Print and shaded views of the part. All mm, measured from the part's lowest x, y and z. Give positions to 0.01 mm unless a question says otherwise; leave off trailing zeros. Loops run counter-clockwise (first coordinate to the right, second up) from the corner with the lowest first, then second, coordinate; pieces in that order, holes last.
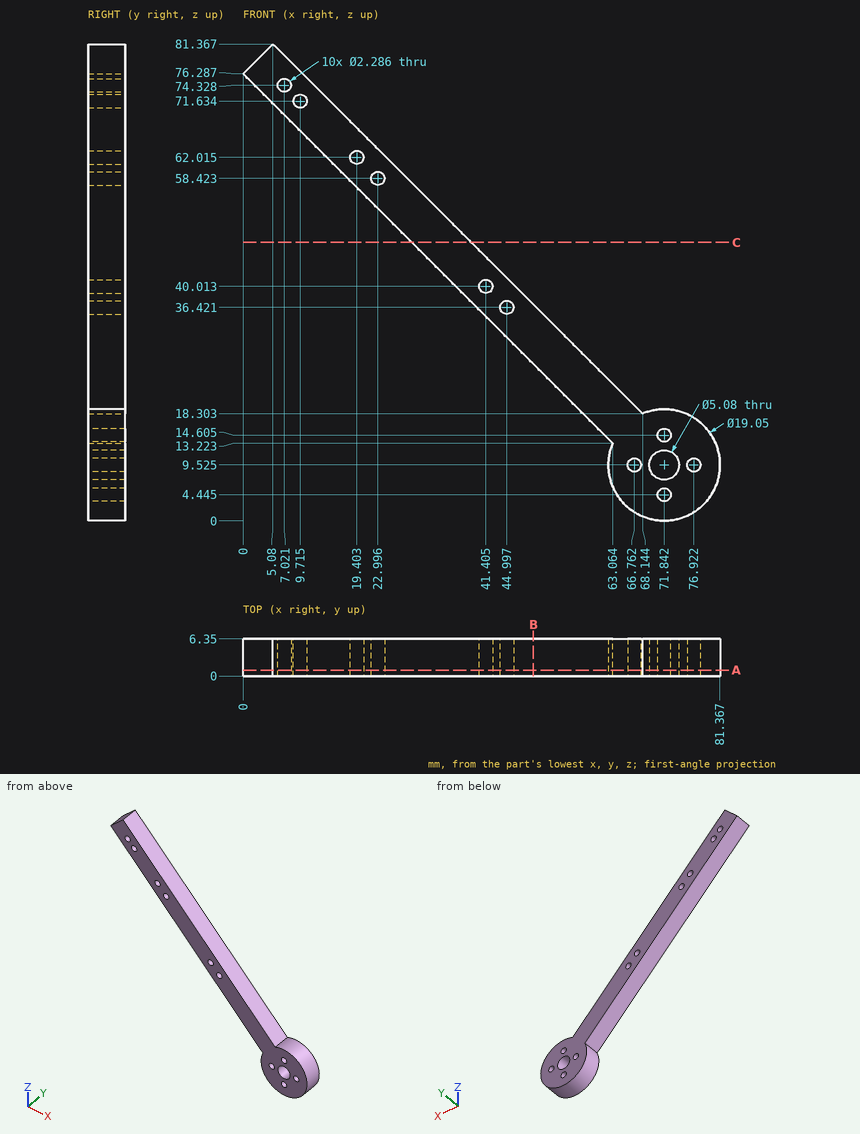
1. Probe line 1 along X through (y, z) = (5.5, 10.5) (1 decimal); line 2 along X through (y, z) = (4, 10) (1 decimal); line 3 along Z through (x, y) = (45, 6) (1 decimal). List the from-to ranges inside material, lowest first.
Responses:
line 1: x = 62.4 to 66.2, 67.4 to 69.5, 74.2 to 76.3, 77.5 to 81.3
line 2: x = 62.3 to 65.7, 67.8 to 69.3, 74.3 to 75.9, 78 to 81.4
line 3: z = 31.3 to 35.3, 37.6 to 41.4
2. Drop flat-ended pins along their axis: pin 1 (3 mm diameter, centred on x = 16, y = 2, fed in from +Z); pin 2 (3 mm diameter, centred on y = 3, z = 55, fed in from -X). Give the stop position or say it passes through.
Responses:
pin 1: stops at z = 71.95
pin 2: stops at x = 19.79
3. Saw through at B-B, the plane x = 49.5. List the corners of the cut face in (y, z).
Responses:
outline: (0, 26.79) - (6.35, 26.79) - (6.35, 36.95) - (0, 36.95) - close
4. Saw through at A-A, the plane y = 1. Count the separate pieces of the cut face and the enclosed holes in it, and give its area (3 significant figures).
Responses:
separate pieces: 1
enclosed holes: 11
area: 861 mm2
5. Saw through at C-C, the plane z = 47.5. List the corners of the cut face in (x, y), and give its area (3 significant figures).
Responses:
outline: (28.79, 0) - (38.95, 0) - (38.95, 6.35) - (28.79, 6.35) - close
area: 64.5 mm2
